Geometry check sheet. Reference: the model listing, model coordinates, mm. Face numbers are marked on the shaded views. A direction names the side the tool comes from. Give positions to 0.01 mm unless a question says otherwise; leave off trailing zeros. Order: outer loops, then holes, each group sorted by start corner. A loop starts at its lowest first (then second) coordinate and runs counter-clockwise, first axis right, second up.
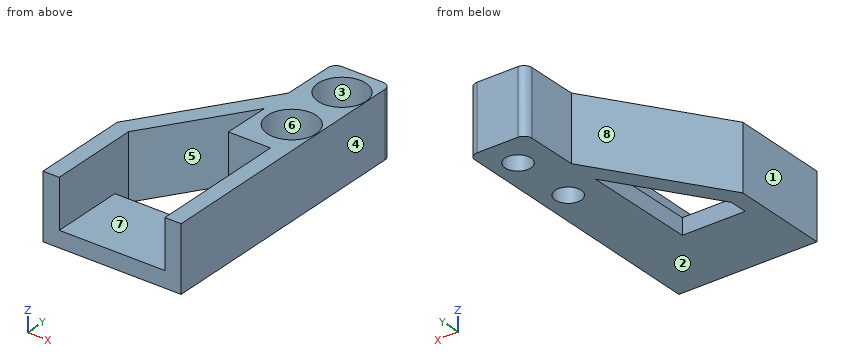
from build123d import *

# Parameters (mm, degrees)
SKETCH_1_R          = 1.6
EXTRUDE_1_DEPTH     = 8
SKETCH_2_W          = 13
SKETCH_2_H          = 17.095287854
CUT_EXTRUDE_1_DEPTH = 6
EXTRUDE_2_DEPTH     = 8
SKETCH_4_R          = 3
SKETCH_4_R_2        = 2.95
CUT_EXTRUDE_2_DEPTH = 3.5
FILLET_1_R          = 1


with BuildPart() as part:
    # 草图1 → 凸台-拉伸1 (new body)
    with BuildSketch(Plane.XY):
        Polygon((0, 0), (6, 0), (6, 24), (6, 34.003436918), (0, 34.003436918), (-1.010556426, 34.003436918), (-1.260244026, 9), (-11, 9), (-11, 0), align=None)
        with Locations((2.89726379, 22)):
            Circle(SKETCH_1_R, mode=Mode.SUBTRACT)
        with Locations((3, 30)):
            Circle(SKETCH_1_R, mode=Mode.SUBTRACT)
    extrude(amount=EXTRUDE_1_DEPTH)

    # 草图2 → 切除-拉伸1 (cut)
    with BuildSketch(Plane.XY.offset(8)):
        with Locations((-2.498171462, 8.547643927)):
            Rectangle(SKETCH_2_W, SKETCH_2_H)
    extrude(amount=-CUT_EXTRUDE_1_DEPTH, mode=Mode.SUBTRACT)

    # 草图3 → 凸台-拉伸2 (add)
    with BuildSketch(Plane.XY.offset(8)):
        Polygon((-11, 12), (-1.083308234, 26.718152327), (-1.121520842, 22.891584471), (-8.998171462, 11.201219742), (-8.998171462, 9), (-11, 9), align=None)
    extrude(amount=-EXTRUDE_2_DEPTH)

    # 草图4 → 切除-拉伸2 (cut)
    with BuildSketch(Plane.XY.offset(8)):
        with Locations((2.89726379, 22)):
            Circle(SKETCH_4_R)
        with Locations((3, 30)):
            Circle(SKETCH_4_R_2)
    extrude(amount=-CUT_EXTRUDE_2_DEPTH, mode=Mode.SUBTRACT)

    # 圆角1
    fillet_1_edges = [part.edges().sort_by_distance(p)[0] for p in [
        (-1.010556426, 34.003436918, 4),
        (6, 34.003436918, 4),
    ]]
    fillet(fillet_1_edges, radius=FILLET_1_R)


solid = part.part
Item 1: Scan lines: L1, parallel to Y at x = 3, z = 2.35; L2, parallel to Y at x = 3, z = 5.5; L3, parallel to X at y = 4, z = 5.25. Record each from-to range of solid material in increasing order.
Reported:
L1: y = 17.1 to 20.4, 23.6 to 28.4, 31.6 to 34
L2: y = 17.1 to 19, 25 to 27.05, 32.95 to 34
L3: x = -11 to -9, 4 to 6
Item 2: Draft check along X on the marked faces 1, 2 and 3. Enter one of: released by +X, released by -X, zero draft, split by the parting line, or undercut.
Reported:
face 1: released by -X
face 2: zero draft
face 3: undercut
Item 3: Sectioned sample at D-D (y = 8). Enter the section's corners in (x, z), and give its area (3 significant figures).
Reported:
outline: (-11, 0) - (6, 0) - (6, 8) - (4, 8) - (4, 2) - (-9, 2) - (-9, 8) - (-11, 8) - close
area: 58.0 mm2
Item 4: Set-up check for the marked faces 4, 5, 6, 7 and 8: record each of +Z, -Z, +X, -X, +Y, -Y from which the full face is reachable in a straight line by a thin tool's end or side.
Reported:
face 4: +Z, -Z, +X, +Y, -Y
face 5: +Z, -Z
face 6: +Z
face 7: +Z, -Y
face 8: +Z, -Z, -X, +Y
Item 5: Sectioned sample at C-C (x = -4.5). Enter the section's corners in (y, z).
Reported:
outline: (0, 0) - (9, 0) - (9, 2) - (0, 2) - close; (17.88, 0) - (21.65, 0) - (21.65, 8) - (17.88, 8) - close
Item 6: Gauge pin test, flat ends, axial feed: pin 1 (1.9 mm diameter, centred on x = 3, y = 30, fed in from -Z); pin 2 (3.5 mm diameter, centred on x = 2.9, y = 22, fed in from +Z); pin 3 (1.5 mm diameter, centred on x = -9, z = 5.5, fed in from +Y); pin 4 (1 mm diameter, centred on x = -6, z = 1.5, fed in from +Y). Record the tip position at first contact, or that the pin passes through.
Reported:
pin 1: passes through
pin 2: stops at z = 4.5
pin 3: stops at y = 16.08
pin 4: stops at y = 20.16
Item 7: Sectioned sample at A-A (z = 5). Enter the section's corners in (x, y).
Reported:
outline: (-11, 0) - (-9, 0) - (-9, 11.2) - (-1.12, 22.89) - (-1.18, 17.1) - (4, 17.1) - (4, 0) - (6, 0) - (6, 33) arc R1 ccw to (5, 34) - (-0.02, 34) arc R1 ccw to (-1.02, 33.01) - (-1.08, 26.72) - (-11, 12) - close; hole circle Ø6 at (2.9, 22); hole circle Ø5.9 at (3, 30)
Item 8: Sectioned sample at B-B (y = 15). Enter the section's corners in (x, z).
Reported:
outline: (-8.98, 0) - (-6.44, 0) - (-6.44, 8) - (-8.98, 8) - close; (-1.2, 0) - (6, 0) - (6, 8) - (4, 8) - (4, 2) - (-1.2, 2) - close
